For this review, take the finished solid that the model builds, in its own axes (mm). A direction names the side the tool comes from. Coordinates: 2 decimals unless noted, no trailing zeros. Loops run counter-clockwise (first coordinate to the right, second up) from the corner with the lowest first, then second, coordinate; pieces in that order, holes last. Notation, with made-up numbers: (-2.75, 55) - (23.25, 55) arc R17 cw to (23.25, 68) - close; hole circle Ø11 at (62.5, 4). An arc over 180 degrees is marked (long way). One line per item, written item: value. Start each with the question number.
1. Take a section at B-B, the plane x = -7.75. State the section outline as (y, z) points, and give its area (3 significant figures).
2. For faces 5 (the face through (1.354, 5, 10)), 6 (the face through (-2.824, 4.93, 7.417)), list the 3-axis set-ups (+Z, -Z, +X, -X, +Y, -Y) from which the entire face can be reached by the end or side of a thin tool; tool diameter is ignored.
3. Take a section at A-A, the plane y = 5.5. State the section outline as (x, z) points.
4. Take a section at C-C, the plane z = 8. State the section outline as (x, y) points, and give its area (3 significant figures).
5. To check wall thickness, follow line 1 (Z direction, x = -4.25, y = 9.5); line 2 (Z direction, x = -3, y = 3.75); line 3 (X direction, y = 1.5, z = 7.75). State the ranges of each line that lie inside material, in increasing order. Write a range as from..to.
6. The part is to be moulded in two halves that separate along Z. For faces 1 (the face through (-4, 5, 17.944)), 2 (the face through (-8.75, 5, 10)), 3 (the face through (-4, 5, 2.667)), 4 (the face through (-6.89, 4.93, 9.17)), say which applies: released by +Z, released by -Z, zero draft, split by the parting line, or undercut.
Autodesk Inventor part; units mm, degrees
ref_plane "YZ Plane" through (0, 0, 0) normal (1, 0, 0) x (0, 1, 0)
ref_plane "XZ Plane" through (0, 0, 0) normal (0, 1, 0) x (-1, 0, 0)
ref_plane "XY Plane" through (0, 0, 0) normal (0, 0, 1) x (1, 0, 0)
sketch "Sketch1" plane through (0, 0, 0) normal (0, 1, 0) x (-1, 0, 0)
  line L0 (8.7498, 17.9442) -> (-1.3539, 17.9442)
  line L1 (-1.3539, 17.9442) -> (-1.3539, 2.6674)
  line L2 (-1.3539, 2.6674) -> (8.7498, 2.6674)
  line L3 (8.7498, 2.6674) -> (8.7498, 17.9442)
  line L4 (6.0139, 5.7417) -> (3.698, 10.8481) construction
  line L5 (8.0291, 6.6557) -> (5.7132, 11.7621)
  line L6 (1.6827, 9.9341) -> (3.9986, 4.8277)
  arc A0 (3.9986, 4.8277) -> (8.0291, 6.6557) centre (6.0139, 5.7417) ccw
  arc A1 (5.7132, 11.7621) -> (1.6827, 9.9341) centre (3.698, 10.8481) ccw
  point P0 (0, 0)
  point P1 (4.8559, 8.2949)
extrude "Extrusion1" add sketch "Sketch1" along normal blind 10
Solutions:
1. outline: (0, 2.67) - (10, 2.67) - (10, 4.37) - (0, 4.37) - close; (0, 7.27) - (10, 7.27) - (10, 17.94) - (0, 17.94) - close
1. area: 124 mm2
2. face 5: +Z, -Z, +X, +Y, -Y
2. face 6: +Y, -Y
3. outline: (-8.75, 2.67) - (1.35, 2.67) - (1.35, 17.94) - (-8.75, 17.94) - close; hole (-8.03, 6.66) arc R2.21 ccw to (-4, 4.83) - (-1.68, 9.93) arc R2.21 ccw to (-5.71, 11.76) - close
4. outline: (-8.75, 0) - (-7.42, 0) - (-7.42, 10) - (-8.75, 10) - close; (-2.56, 0) - (1.35, 0) - (1.35, 10) - (-2.56, 10) - close
4. area: 52.4 mm2
5. line 1: 2.67..4.41, 12.99..17.94
5. line 2: 2.67..7.03, 12.95..17.94
5. line 3: -8.75..-7.53, -2.67..1.35
6. face 1: released by +Z
6. face 2: zero draft
6. face 3: released by -Z
6. face 4: undercut
